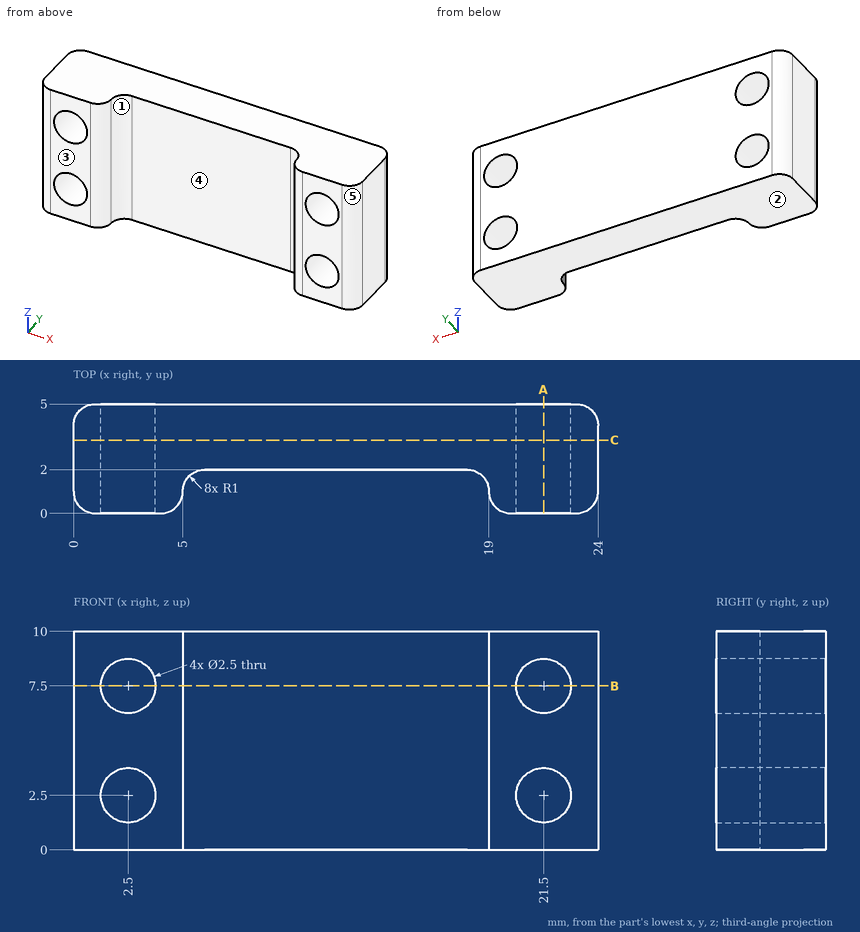
Print and shaded views of the part. All mm, measured from the part's lowest x, y and z. A direction names the side the tool comes from. Coordinates: 2 decimals unless noted, no trailing zeros. Write each loop counter-clockwise with the first axis right and the second up, starting at its lowest first coordinate (ties: lowest second). Pieces come first, ordered by that corner, then holes. Notation, with made-up numbers: (82, 54) -> (128, 54) arc R31 cw to (128, 82) -> close; hole circle Ø7 at (-27, 21). An arc over 180 degrees is marked (long way). Use CSV: the item, a comma, the result in double quotes. Start each with the question number.
Q1. Cut at A-A, the plane x = 21.5. List the corners of the cut face in (y, z), then the cut area to 3 significant figures.
Q2. 3-axis set-ups, long thin cutter, end or side, ignore diameter. For the marked faces 1 and 2: which of +Z, -Z, +X, -X, +Y, -Y reach the whole face in a straight line?
Q3. Drill centre lines: probe 1 along X at (y, z) = (2.6, 2.5); probe 2 along X at (y, z) = (0.9, 6) (3 decimals); probe 3 along X at (y, z) = (1.75, 2.5). Where is each one in solid material? Low to high.
Q4. Flat gauge pins, fed straight in: pin 1 Ø1 at (x, z) = (19, 3.5) entering from -Y; pin 2 Ø3 at (x, z) = (14.5, 2.5) entering from -Y. Where does each tip first touch, or does it go through?
Q5. Cut at C-C, the plane y = 3.35. List the corners of the cut face in (x, z).
Q6. Cut at B-B, the plane z = 7.5. State how many separate pieces and enclosed holes the cut face has.
Q7. Pull direction X, two halves, no side cores. Call the marked faces 3, 4 and 5: released by +X, released by -X, zero draft, split by the parting line, or undercut.
Checked values:
1,outline,"(0, 0) -> (5, 0) -> (5, 1.25) -> (0, 1.25) -> close; (0, 3.75) -> (5, 3.75) -> (5, 6.25) -> (0, 6.25) -> close; (0, 8.75) -> (5, 8.75) -> (5, 10) -> (0, 10) -> close"
1,area,"25.0 mm²"
2,face 1,"+Z, -Z, -Y"
2,face 2,"-Z, +X, -X, +Y, -Y"
3,probe 1,"x = 0 to 1.25, 3.75 to 20.25, 22.75 to 24"
3,probe 2,"x = 0.005 to 4.995, 19.005 to 23.995"
3,probe 3,"x = 0 to 1.25, 3.75 to 5.34, 18.66 to 20.25, 22.75 to 24"
4,pin 1,"stops at y = 0.13"
4,pin 2,"stops at y = 2"
5,outline,"(0, 0) -> (24, 0) -> (24, 10) -> (0, 10) -> close; hole circle Ø2.5 at (2.5, 2.5); hole circle Ø2.5 at (2.5, 7.5); hole circle Ø2.5 at (21.5, 2.5); hole circle Ø2.5 at (21.5, 7.5)"
6,separate pieces,"3"
6,enclosed holes,"0"
7,face 3,"zero draft"
7,face 4,"undercut"
7,face 5,"released by +X"
